from build123d import *

# Parameters (mm, degrees)
SKETCH1_W           = 44.8
SKETCH1_H           = 19.8
BOSS_EXTRUDE1_DEPTH = 5
SKETCH2_R           = 1.1
CUT_EXTRUDE1_DEPTH  = 13
SKETCH3_R           = 1.5
CUT_EXTRUDE2_DEPTH  = 10
SKETCH4_W           = 21
SKETCH4_H           = 12
CUT_EXTRUDE3_DEPTH  = 10
FILLET1_START       = 9.18
FILLET1_DEPTH       = 19.8
BOSS_EXTRUDE2_START = -5
SKETCH5_R           = 3.5
SKETCH5_R_2         = 1.5
BOSS_EXTRUDE2_DEPTH = 5
FILLET2_R           = 0.5


with BuildPart() as part:
    # Sketch1 → Boss-Extrude1 (new body)
    with BuildSketch(Plane.XY):
        with Locations((0, 19.08)):
            Rectangle(SKETCH1_W, SKETCH1_H)
    extrude(amount=BOSS_EXTRUDE1_DEPTH)

    # Sketch2 → Cut-Extrude1 (cut)
    with BuildSketch(Plane.XY.offset(5)):
        with Locations((-20, 25)):
            Circle(SKETCH2_R)
        with Locations((-20, 13)):
            Circle(SKETCH2_R)
        with Locations((20, 25)):
            Circle(SKETCH2_R)
        with Locations((20, 13)):
            Circle(SKETCH2_R)
    extrude(amount=-CUT_EXTRUDE1_DEPTH, mode=Mode.SUBTRACT)

    # Sketch3 → Cut-Extrude2 (cut)
    with BuildSketch(Plane.XY.offset(5)):
        with Locations((-14, 19)):
            Circle(SKETCH3_R)
        with Locations((14, 19)):
            Circle(SKETCH3_R)
    extrude(amount=-CUT_EXTRUDE2_DEPTH, mode=Mode.SUBTRACT)

    # Sketch4 → Cut-Extrude3 (cut)
    with BuildSketch(Plane.XY.offset(5)):
        with Locations((0, 19)):
            Rectangle(SKETCH4_W, SKETCH4_H)
    extrude(amount=-CUT_EXTRUDE3_DEPTH, mode=Mode.SUBTRACT)

    # Fillet1: read off the stored shape, not the designer's step
    # Fillet1 outline → Fillet1 (cut)
    with BuildSketch(Plane(origin=(0, 0, 0), x_dir=(1, 0, 0), z_dir=(0, 1, 0)).offset(FILLET1_START)):
        with BuildLine():
            Line((22.4, -5), (22.4, 0))
            ThreePointArc((22.4, 0), (14.477130086, -3.722813233), (5.816876048, -5))
            Line((5.816876048, -5), (22.4, -5))
        make_face()
        with BuildLine():
            Line((-22.4, -5), (-5.816876048, -5))
            ThreePointArc((-5.816876048, -5), (-14.477130086, -3.722813233), (-22.4, 0))
            Line((-22.4, 0), (-22.4, -5))
        make_face()
    extrude(amount=FILLET1_DEPTH, mode=Mode.SUBTRACT)

    # Sketch5 → Boss-Extrude2 (add)
    # profile 1 of 6: a face of its own
    with BuildSketch(Plane(origin=(0, 0, 0), x_dir=(-1, 0, 0), z_dir=(0, 0, -1)).offset(BOSS_EXTRUDE2_START)):
        with Locations((-14, 19)):
            Circle(SKETCH5_R)
        with Locations((-14, 19)):
            Circle(SKETCH5_R_2, mode=Mode.SUBTRACT)
    # profile 2 of 6: a face of its own
    with BuildSketch(Plane(origin=(0, 0, 0), x_dir=(-1, 0, 0), z_dir=(0, 0, -1)).offset(BOSS_EXTRUDE2_START)):
        with BuildLine():
            Line((-10.5, 22.5), (-14, 22.5))
            ThreePointArc((-14, 22.5), (-11.525126266, 21.474873734), (-10.5, 19))
            Line((-10.5, 19), (-10.5, 22.5))
        make_face()
    # profile 3 of 6: a face of its own
    with BuildSketch(Plane(origin=(0, 0, 0), x_dir=(-1, 0, 0), z_dir=(0, 0, -1)).offset(BOSS_EXTRUDE2_START)):
        with BuildLine():
            Line((-10.5, 15.5), (-10.5, 19))
            ThreePointArc((-10.5, 19), (-11.525126266, 16.525126266), (-14, 15.5))
            Line((-14, 15.5), (-10.5, 15.5))
        make_face()
    # profile 4 of 6: a face of its own
    with BuildSketch(Plane(origin=(0, 0, 0), x_dir=(-1, 0, 0), z_dir=(0, 0, -1)).offset(BOSS_EXTRUDE2_START)):
        with Locations((14, 19)):
            Circle(SKETCH5_R)
        with Locations((14, 19)):
            Circle(SKETCH5_R_2, mode=Mode.SUBTRACT)
    # profile 5 of 6: a face of its own
    with BuildSketch(Plane(origin=(0, 0, 0), x_dir=(-1, 0, 0), z_dir=(0, 0, -1)).offset(BOSS_EXTRUDE2_START)):
        with BuildLine():
            ThreePointArc((14, 15.5), (11.525126266, 16.525126266), (10.5, 19))
            Line((10.5, 19), (10.5, 15.5))
            Line((10.5, 15.5), (14, 15.5))
        make_face()
    # profile 6 of 6: a face of its own
    with BuildSketch(Plane(origin=(0, 0, 0), x_dir=(-1, 0, 0), z_dir=(0, 0, -1)).offset(BOSS_EXTRUDE2_START)):
        with BuildLine():
            ThreePointArc((10.5, 19), (11.525126266, 21.474873734), (14, 22.5))
            Line((14, 22.5), (10.5, 22.5))
            Line((10.5, 22.5), (10.5, 19))
        make_face()
    extrude(amount=BOSS_EXTRUDE2_DEPTH)

    # Fillet2
    fillet2_edges = [part.edges().sort_by_distance(p)[0] for p in [
        (-10.5, 13, 2.316109055),
        (-10.5, 25, 2.316109055),
        (10.5, 25, 2.316109055),
        (10.5, 13, 2.316109055),
    ]]
    fillet(fillet2_edges, radius=FILLET2_R)


solid = part.part
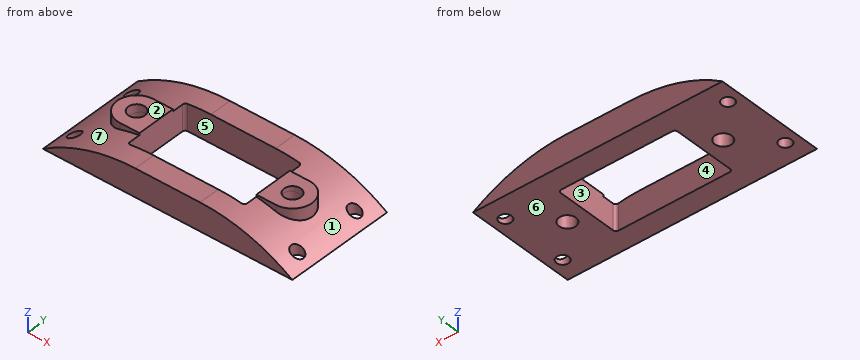
Here's how the part is built. I have some questions about the finished solid (model axes, mm). Face numbers are marked on the shaded views. A direction names the side the tool comes from. Coordinates: 2 decimals unless noted, no trailing zeros. Order: outer loops, then holes, each group sorted by start corner. A loop starts at its lowest first (then second) coordinate and runs counter-clockwise, first axis right, second up. Notation, with made-up numbers: (-9.5, 5) - (-1.5, 5) arc R31 ccw to (-1.5, 36) - close; hole circle Ø1 at (80, 23). An arc over 180 degrees is marked (long way). Use CSV: the item, a comma, the result in double quotes. Start each with the question number.
1. If we mould it in two halves opening along X, with no side actions, what happens to the marked faces 1, 2, 3 and 4? For each: +X half, -X half, draft (parallel to the pull), parting line (faces both ways), or undercut.
2. Suppose I cut it at C-C on z = 1.45. List the corners of the cut face in (x, y) for me.
3. Please list where these lines run through material, in increasing order: line 1 (Y direction, x = 20, z = 1.35); line 2 (X direction, y = 19, z = 3.75); line 3 (Y direction, x = -10, z = 0.4). Write a range as from..to.
4. I'm going to push flat-ended pins straight in: pin 1 (2 mm diameter, centred on y = 15, z = 3, fed in from -X); pin 2 (2.5 mm diameter, centred on x = -14, y = 19, fed in from -Z). Where does each tip first touch, or does it pass through?
5. Suppose I cut it at D-D on y = 17. List the corners of the cut face in (x, z) for me.
6. Suppose I cut it at A-A on y = 19. List the corners of the cut face in (x, z) for me.
7. Suppose I cut it at B-B on x = 0.5. List the corners of the cut face in (y, z) for me.
8. For the marked faces 5, 6 and 7, which set-ups out of +Z, -Z, +X, -X, +Y, -Y let a thin tool reach every point of the face, with its end or its side?
Output:
1,face 1,"+X half"
1,face 2,"draft"
1,face 3,"undercut"
1,face 4,"undercut"
2,outline,"(-19.97, 9.18) - (19.97, 9.18) - (19.97, 11.9) arc R1.1 cw to (19.97, 14.1) - (19.97, 23.9) arc R1.1 cw to (19.97, 26.1) - (19.97, 28.98) - (-19.97, 28.98) - (-19.97, 26.1) arc R1.1 cw to (-19.97, 23.9) - (-19.97, 14.1) arc R1.1 cw to (-19.97, 11.9) - close; hole circle Ø3 at (-14, 19); hole (-10.5, 13.5) arc R0.5 ccw to (-10, 13) - (10, 13) arc R0.5 ccw to (10.5, 13.5) - (10.5, 24.5) arc R0.5 ccw to (10, 25) - (-10, 25) arc R0.5 ccw to (-10.5, 24.5) - close; hole circle Ø3 at (14, 19)"
3,line 1,"y = 9.18..11.9, 14.1..23.9, 26.1..28.98"
3,line 2,"x = -17.5..-15.5, -12.5..-10.5, 10.5..12.5, 15.5..17.5"
3,line 3,"y = 9.18..13, 25..28.98"
4,pin 1,"stops at x = -18.89"
4,pin 2,"passes through"
5,outline,"(-22.4, 0) - (-10.5, 0) - (-10.5, 5) - (-16.87, 5) - (-16.87, 2.89) arc R30 ccw to start; (10.5, 0) - (22.4, 0) arc R30 ccw to (16.87, 2.89) - (16.87, 5) - (10.5, 5) - close"
6,outline,"(-22.4, 0) - (-15.5, 0) - (-15.5, 5) - (-17.5, 5) - (-17.5, 2.63) arc R30 ccw to start; (-12.5, 0) - (-10.5, 0) - (-10.5, 5) - (-12.5, 5) - close; (10.5, 0) - (12.5, 0) - (12.5, 5) - (10.5, 5) - close; (15.5, 0) - (22.4, 0) arc R30 ccw to (17.5, 2.63) - (17.5, 5) - (15.5, 5) - close"
7,outline,"(9.18, 0) - (13, 0) - (13, 5) - (9.18, 5) - close; (25, 0) - (28.98, 0) - (28.98, 5) - (25, 5) - close"
8,face 5,"+Z, -Z"
8,face 6,"-Z, +X, -X, +Y, -Y"
8,face 7,"+Z, -X"
